Read the model definition and answer for the solid it produces. Units are mm, in the model's axes. Coordinates: 2 decimals unless noted, no trailing zeros. Loops run counter-clockwise (first coordinate to the right, second up) from the corner with the lowest first, then second, coordinate; pieces in that order, holes last. Notation, with made-up numbers: (3.5, 1) - (20.5, 1) arc R15 cw to (20.5, 11) - close; hole circle Ø7 at (56.5, 67.5). An arc over 180 degrees is marked (long way). Use one line per item in the form item = value. Start each with the question number.
1) Consider line 1 (X direction, y = 0.45, z = 0); line 2 (Z direction, x = -14.5, y = 0.4). Determine where each line is inside the solid, lowest interval first.
2) A cutting plane is placed at B-B (z = 0). Give the vertices of the cut face in (x, y).
3) A cutting plane is placed at A-A (x = -13.75). Give the vertices of the cut face in (y, z).
4) The mould has two halves that part along X. Classify faces 1 (the face through (-14.726, 0.507, -0.217)), 2 (the face through (17.95, 0.5, 0.1)), 3 (the face through (0, 1, 0)), 4 (the face through (12.774, 0.507, -0.217)): released by +X, released by -X, zero draft, split by the parting line, or undercut.
5) This flat-tipped pin is pushed along its axis until it touches: P1, Ø1.8, axis at x = -13.75, z = 0, coming from the -Y side. Where does it stop, or does it pass through?
from build123d import *

# Parameters (mm, degrees)
ESBO_O1_W                = 35.9
ESBO_O1_H                = 20
RESSALTO_EXTRUS_O1_DEPTH = 1
CORTE_EXTRUS_O1_REACH    = 22.572
ESBO_O2_R                = 1


with BuildPart() as part:
    # Esboço1 → Ressalto-extrusão1 (new body)
    with BuildSketch(Plane(origin=(0, 0, 0), x_dir=(1, 0, 0), z_dir=(0, 1, 0))):
        Rectangle(ESBO_O1_W, ESBO_O1_H)
    extrude(amount=RESSALTO_EXTRUS_O1_DEPTH)

    # Esboço2 → Corte-extrusão1 (cut, up to next)
    with BuildSketch(Plane(origin=(0, 1, 0), x_dir=(1, 0, 0), z_dir=(0, 1, 0)), mode=Mode.PRIVATE) as corte_extrus_o1_sk1:
        with Locations(Location((13.75, 0, 0), (0, 0, 270))):
            Circle(ESBO_O2_R)
    corte_extrus_o1_tool1 = extrude(corte_extrus_o1_sk1.sketch, amount=-CORTE_EXTRUS_O1_REACH, mode=Mode.PRIVATE) & part.part
    # Esboço2 → Corte-extrusão1 (cut, up to next)
    with BuildSketch(Plane(origin=(0, 1, 0), x_dir=(1, 0, 0), z_dir=(0, 1, 0)), mode=Mode.PRIVATE) as corte_extrus_o1_sk2:
        with Locations(Location((-13.75, 0, 0), (0, 0, 270))):
            Circle(ESBO_O2_R)
    corte_extrus_o1_tool2 = extrude(corte_extrus_o1_sk2.sketch, amount=-CORTE_EXTRUS_O1_REACH, mode=Mode.PRIVATE) & part.part
    add(corte_extrus_o1_tool1.solids().sort_by_distance((13.75, 1, 0))[0], mode=Mode.SUBTRACT)
    add(corte_extrus_o1_tool2.solids().sort_by_distance((-13.75, 1, 0))[0], mode=Mode.SUBTRACT)


solid = part.part
Found:
q1.line_1 = -17.95 to -14.75, -12.75 to 12.75, 14.75 to 17.95
q1.line_2 = -10 to -0.66, 0.66 to 10
q2.outline = (-17.95, 0) - (-14.75, 0) - (-14.75, 1) - (-17.95, 1) - close; (-12.75, 0) - (12.75, 0) - (12.75, 1) - (-12.75, 1) - close; (14.75, 0) - (17.95, 0) - (17.95, 1) - (14.75, 1) - close
q3.outline = (0, -10) - (1, -10) - (1, -1) - (0, -1) - close; (0, 1) - (1, 1) - (1, 10) - (0, 10) - close
q4.face_1 = undercut
q4.face_2 = released by +X
q4.face_3 = zero draft
q4.face_4 = undercut
q5.P1 = through
